from build123d import *

# Parameters (mm, degrees)
BOSS_EXTRUDE1_DEPTH = 8
BOSS_EXTRUDE2_DEPTH = 5
SKETCH3_R           = 2.75
CUT_EXTRUDE1_DEPTH  = 36.813646862
FILLET1_R           = 1
CUT_EXTRUDE2_DEPTH  = 3
SKETCH5_R           = 6.6
CUT_EXTRUDE3_DEPTH  = 2
SKETCH6_R           = 4.5
CUT_EXTRUDE4_DEPTH  = 36.137121418


with BuildPart() as part:
    # Sketch1 → Boss-Extrude1 (new body)
    with BuildSketch(Plane(origin=(0, 0, 0), x_dir=(1, 0, 0), z_dir=(0, 1, 0))):
        with BuildLine():
            Line((24.015632569, -4.149601491), (-1.78233066, -4.083471877))
            ThreePointArc((-1.78233066, -4.083471877), (-9.26308084, 3.435728662), (-1.743880301, 10.916478842))
            Line((-1.743880301, 10.916478842), (24.054082929, 10.850349227))
            ThreePointArc((24.054082929, 10.850349227), (31.534833108, 3.331148688), (24.015632569, -4.149601491))
        make_face()
    extrude(amount=BOSS_EXTRUDE1_DEPTH)

    # Sketch2 → Boss-Extrude2 (add)
    with BuildSketch(Plane(origin=(0, 8, 0), x_dir=(1, 0, 0), z_dir=(0, 1, 0))):
        Polygon((-3.25175247, -0.833664766), (1.173324698, 0.002213248), (2.661971688, 4.252381497), (-0.274458491, 7.666671731), (-4.69953566, 6.830793717), (-6.188182649, 2.580625468), align=None)
    extrude(amount=BOSS_EXTRUDE2_DEPTH)

    # Sketch3 → Cut-Extrude1 (cut, through all)
    with BuildSketch(Plane(origin=(0, 13, 0), x_dir=(1, 0, 0), z_dir=(0, 1, 0))):
        with Locations(Location((-1.763105481, 3.416503482, 0), (0, 0, 270))):
            Circle(SKETCH3_R)
    extrude(amount=-CUT_EXTRUDE1_DEPTH, mode=Mode.SUBTRACT)

    # Fillet1
    fillet1_edges = [part.edges().sort_by_distance(p)[0] for p in [
        (-6.188182649, 10.5, -2.580625468),
        (-3.25175247, 10.5, 0.833664766),
        (1.173324698, 10.5, -0.002213248),
        (2.661971688, 10.5, -4.252381497),
        (-0.274458491, 10.5, -7.666671731),
        (-4.69953566, 10.5, -6.830793717),
    ]]
    fillet(fillet1_edges, radius=FILLET1_R)

    # Sketch4 → Cut-Extrude2 (cut)
    with BuildSketch(Plane.XZ):
        with BuildLine():
            Line((2.943011006, -3.542205297), (1.836068373, -0.381823779))
            ThreePointArc((1.836068373, -0.381823779), (1.398479703, 0.259582363), (0.698813727, 0.596262041))
            Line((0.698813727, 0.596262041), (-2.59162827, 1.217812359))
            ThreePointArc((-2.59162827, 1.217812359), (-3.365896618, 1.159552526), (-4.00730276, 0.721963855))
            Line((-4.00730276, 0.721963855), (-6.190802123, -1.816867345))
            ThreePointArc((-6.190802123, -1.816867345), (-6.527481801, -2.51653332), (-6.469221968, -3.290801668))
            Line((-6.469221968, -3.290801668), (-5.362279334, -6.451183186))
            ThreePointArc((-5.362279334, -6.451183186), (-4.924690664, -7.092589328), (-4.225024689, -7.429269006))
            Line((-4.225024689, -7.429269006), (-0.934582692, -8.050819324))
            ThreePointArc((-0.934582692, -8.050819324), (-0.160314344, -7.99255949), (0.481091798, -7.55497082))
            Line((0.481091798, -7.55497082), (2.664591162, -5.01613962))
            ThreePointArc((2.664591162, -5.01613962), (3.00127084, -4.316473645), (2.943011006, -3.542205297))
        make_face()
    extrude(amount=-CUT_EXTRUDE2_DEPTH, mode=Mode.SUBTRACT)

    # Sketch5 → Cut-Extrude3 (cut)
    with BuildSketch(Plane.XZ):
        with Locations(Location((24.034857749, -3.350373868, 0), (0, 0, 270))):
            Circle(SKETCH5_R)
    extrude(amount=-CUT_EXTRUDE3_DEPTH, mode=Mode.SUBTRACT)

    # Sketch6 → Cut-Extrude4 (cut, through all)
    with BuildSketch(Plane.XZ.offset(-2)):
        with Locations(Location((24.034857749, -3.350373868, 0), (0, 0, 270))):
            Circle(SKETCH6_R)
    extrude(amount=-CUT_EXTRUDE4_DEPTH, mode=Mode.SUBTRACT)


solid = part.part
For this review, take the finished solid that the model builds, in its own axes (mm). A direction names the side the tool comes from. Give positions to 0.01 mm unless a question says otherwise; leave off trailing zeros. Loops run counter-clockwise (first coordinate to the right, second up) from the corner with the lowest first, then second, coordinate; pieces in that order, holes last.
Item 1: Take a section at C-C, the plane z = 1.75. State the section outline as (x, y) points, and give its area (3 significant figures).
Item 2: Take a section at B-B, the plane y = 10. State the section outline as (x, z) points.
Item 3: Tool access review of faces 5 (the cylindrical face through (-0.333, 10.535, -7.523)), 6 (the flat face through (-2.603, 1.479, -7.736)), 7 (the flat face through (-4.735, 10.465, -0.891)): name each direction out of +Z, -Z, +X, -X, +Y, -Y from which nothing blocks a thin tool from reaching the whole face with its end or side.
Item 4: Take a section at D-D, the plane x = 19. State the section outline as (y, z) points, and give its area (3 significant figures).
Item 5: Draft analysis for pull direction Z (two halves, no side actions). For faces 1 (the cylindrical face through (-3.36, 1.48, 1.16)), 2 (the cylindrical face through (-9.26, 3.94, -3.27)), 3 (the cylindrical face through (-6.525, 1.479, -2.506)), 4 (the flat face through (1.91, 10.46, -2.11)), state which applies: +Z half, -Z half, draft (parallel to the pull), parting line (faces both ways), or undercut.
Item 6: Insertion check: pin 1 (6 mm diameter, centred on y = 9, z = 0.5, fed in from -X); pin 2 (1 mm diameter, centred on x = 20.5, z = -6.5, fed in from +Y); pin 3 (3 mm diameter, centred on x = 22.5, z = -5.5, fed in from +Y); pin 4 (3 mm diameter, centred on x = -4, z = -4, fed in from -Y). Each pin has a flat end and moves straight along its axis. Give the tip position at first contact, or say it passes through.
Item 7: For line 1 along X through (y, z) = (2.25, -6); line 2 along X through (y, z) = (2.25, -3.75); line 3 along X through (y, z) = (8.25, -3.25), list the stretches that pass through material, from the lowest coordinate up.
Item 8: Take a section at A-A, the plane x = 26. State the section outline as (y, z) points, and give its area (3 significant figures).
Calculated:
1. outline: (-7.2, 0) - (19.85, 0) - (19.85, 2) - (28.22, 2) - (28.22, 0) - (29.53, 0) - (29.53, 8) - (-7.2, 8) - close
1. area: 277 mm2
2. outline: (-6, -3.13) - (-4.89, -6.29) arc R1 ccw to (-4.13, -6.94) - (-0.84, -7.56) arc R1 ccw to (0.1, -7.23) - (2.29, -4.69) arc R1 ccw to (2.47, -3.71) - (1.36, -0.55) arc R1 ccw to (0.61, 0.1) - (-2.68, 0.73) arc R1 ccw to (-3.63, 0.4) - (-5.81, -2.14) arc R1 ccw to start; hole circle Ø5.5 at (-1.76, -3.42)
3. face 5: -Z, +Y
3. face 6: -Y
3. face 7: +Z, -X, +Y
4. outline: (0, -10.86) - (8, -10.86) - (8, 4.14) - (0, 4.14) - (0, 0.92) - (2, 0.92) - (2, -7.62) - (0, -7.62) - close
4. area: 103 mm2
5. face 1: undercut
5. face 2: parting line
5. face 3: undercut
5. face 4: +Z half
6. pin 1: stops at x = -9.18
6. pin 2: stops at y = 8
6. pin 3: passes through
6. pin 4: stops at y = 3
7. line 1: x = -8.8 to -5.52, 1.82 to 20.4, 27.67 to 31.05
7. line 2: x = -9.26 to -6.31, 3 to 19.55, 28.52 to 31.52
7. line 3: x = -5.95 to -4.51, 0.98 to 2.31
8. outline: (0, -10.59) - (8, -10.59) - (8, -7.4) - (2, -7.4) - (2, -9.65) - (0, -9.65) - close; (0, 2.95) - (2, 2.95) - (2, 0.7) - (8, 0.7) - (8, 3.89) - (0, 3.89) - close
8. area: 42.0 mm2
